Autodesk Inventor part; units mm, degrees
ref_plane "YZ Plane" through (0, 0, 0) normal (1, 0, 0) x (0, 1, 0)
ref_plane "XZ Plane" through (0, 0, 0) normal (0, 1, 0) x (-1, 0, 0)
ref_plane "XY Plane" through (0, 0, 0) normal (0, 0, 1) x (1, 0, 0)
sketch "スケッチ1" plane through (0, 0, 0) normal (0, 0, 1) x (1, 0, 0)
  circle A0 centre (0, 0) radius 6.25
  line L0 (0, 13) -> (24, 13)
  line L1 (24, 13) -> (24, -13)
  line L2 (24, -13) -> (0, -13)
  line L3 (0, -13) -> (0, 13)
  line L4 (0, 13) -> (-3, 13)
  line L5 (-3, 13) -> (-3, -13)
  line L6 (-3, -13) -> (0, -13)
  line L7 (0, -13) -> (0, 13)
  line L8 (16, -13) -> (16, -6.25)
  line L9 (16, -6.25) -> (0, -6.25)
  line L10 (-3, -10) -> (24, -10)
  arc A1 (10.75, -6.25) -> (4, -13) centre (10.75, -13) ccw
  line L11 (4, -13) -> (4, -9.651) construction
  point P0 (24, 0)
  point P1 (-3, 5.4829)
  point P2 (-3, -5.4829)
  point P3 (0, 0)
  point P4 (16, -10)
  point P5 (4.7033, -10)
  dimension "d0" = 12.5
  dimension "d1" = 24
  dimension "d2" = 26
  dimension "d3" = 3
  dimension "d5" = 8
  dimension "d16" = 3
  dimension "d17" = 7
extrude "プレート1" add sketch "スケッチ1" along normal blind 1.5 contours L3 L10 L5 A0 | L9 A1 L10 L3 | A0 L3 L0 L1 L10 L8 L9 | L10 A1 L2 L3 | L3 L6 L5 L10 | A0 L5 L4 L3
sketch "スケッチ2" plane through (24, -8.5, 0) normal (0, -1, 0) x (1, 0, 0)
  line L0 (-8, 0) -> (0, 0)
  line L1 (0, 0) -> (0, 11)
  line L2 (0, 11) -> (-8, 11)
  line L3 (-8, 11) -> (-8, 0)
edge flange "フランジ1" height 11 angle 90 thickness 1.5 bend radius 1.5 thickness toward (0, -1, 0) relief tear relief width 1.5 relief depth 0.75 edges at (20, -10, 1.5) wall of the first edge with corners at (16, -8.5, 0) (24, -8.5, 0) (24, -8.5, 11) (16, -8.5, 11)
bend "曲げ1"
corner "コーナー1"
equation "\"d4\" = Thickness"
equation "\"d6\" = BendReliefWidth"
equation "\"d7\" = BendReliefDepth"
equation "\"d8\" = MinimumRemnant"
equation "\"d9\" = TransitionRadius"
equation "\"d12\" = BendRadius"
equation "\"d13\" = CornerReliefSize"
equation "\"d14\" = GapSize"
equation "\"d15\" = JacobiRadiusSize"
equation "\"BendRadius\" = Thickness"
equation "\"BendReliefWidth\" = Thickness"
equation "\"BendReliefDepth\" = 0.5 * Thickness"
equation "\"CornerReliefSize\" = 4 * Thickness"
equation "\"MinimumRemnant\" = 2 * Thickness"
equation "\"TransitionRadius\" = BendRadius"
equation "\"JacobiRadiusSize\" = BendRadius"
equation "\"GapSize\" = Thickness"
properties part number "hipjoint_toleg_under_up_right"
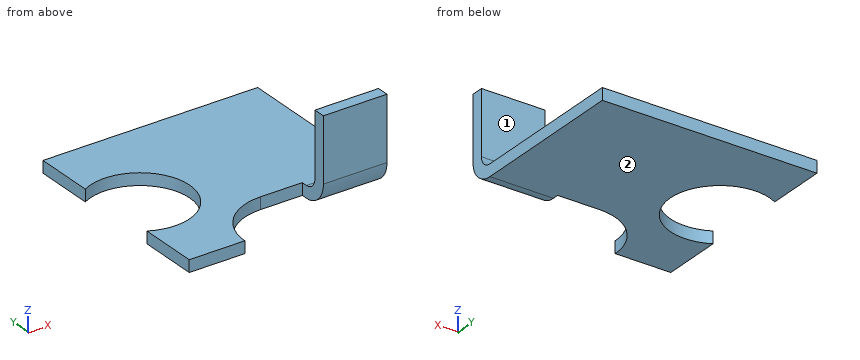
Geometry: final body of the model. Coordinates: model frame, mm. Face numbers are marked on the shaded views. A direction names the side the tool comes from. Coordinates: 2 decimals unless noted, no trailing zeros. Order: outer loops, then holes, each group sorted by start corner. A loop starts at its lowest first (then second) coordinate and runs counter-clockwise, first axis right, second up. Notation, with made-up numbers: (-13, 40) - (6, 40) arc R14 cw to (6, 49) - close; hole circle Ø7 at (-16.75, 47). An arc over 180 degrees is marked (long way). Return JSON: item names as keys, results as strings. Group by question number.
1. Cut plane C-C (y = 9.25). Output: boundary loops of the cut face in (x, z).
2. Cut plane D-D (x = 0). Output: boundary loops of the cut face in (y, z), plus the area to 4 significant figures.
3. Set-up query: the marked faces 1 and 2. Return all of +Z, -Z, +X, -X, +Y, -Y with unobstructed straight access to the full face (end or side cutting, diameter ignored); none if empty.
4. Cut plane A-A (x = 3). Output: boundary loops of the cut face in (y, z).
5. Pin query (flat end, axial travel): pin 1 (3 mm diameter, centred on y = 0, z = 2, fed in from -X); pin 2 (1.5 mm diameter, centred on x = 9, y = 2.5, fed in from +Z); pin 3 (1.2 mm diameter, centred on x = 13, z = 1, fed in from -Y). Return the tip coordinate at first contact, or that it passes through.
6. Cut plane B-B (x = 17.5). Output: boundary loops of the cut face in (y, z).
7. Material intervals for line 1 along Y through (x, z) = (0, 1.05); line 2 along Z through (x, y) = (15.5, -2.5); line 3 along Y through (x, z) = (20, 9.75), sorted ascending. Write a range as [from, to].
Resolved:
{
 "1": {"outline": "(-3, 0) - (24, 0) - (24, 1.5) - (-3, 1.5) - close"},
 "2": {"outline": "(-13, 0) - (-6.25, 0) - (-6.25, 1.5) - (-13, 1.5) - close; (6.25, 0) - (13, 0) - (13, 1.5) - (6.25, 1.5) - close", "area": "20.25 mm²"},
 "3": {"face 1": "+Z, +X, -X, +Y", "face 2": "-Z, +X, -X, +Y, -Y"},
 "4": {"outline": "(-13, 0) - (-5.48, 0) - (-5.48, 1.5) - (-13, 1.5) - close; (5.48, 0) - (13, 0) - (13, 1.5) - (5.48, 1.5) - close"},
 "5": {"pin 1": "stops at x = 6.09", "pin 2": "stops at z = 1.5", "pin 3": "stops at y = -6.25"},
 "6": {"outline": "(-10, 3) arc R3 ccw to (-7, 0) - (13, 0) - (13, 1.5) - (-7, 1.5) arc R1.5 cw to (-8.5, 3) - (-8.5, 11) - (-10, 11) - close"},
 "7": {"line 1": "y = [-13, -6.25], [6.25, 13]", "line 2": "z = [0, 1.5]", "line 3": "y = [-10, -8.5]"}
}
